Read the model definition and answer for the solid it produces. Units are mm, in the model's axes. Round coordinates to 2 decimals unless told otherwise and drop trailing zeros. Write each loop counter-clockwise with the first axis right and the second up, starting at its lowest first coordinate (ties: lowest second). Pieces come first, ordered by that corner, then holes. Notation, with made-up numbers: (62, 31.25) - (80, 31.25) arc R18 ccw to (80, 61.25) - close; hole circle Ø7 at (21, -8). An arc over 180 degrees is marked (long way). Use one line per item in the form item = value. Start each with the question number.
1) Consider line 1 along X through (y, z) = (65, 1); line 2 along X through (y, z) = (47, 3); line 3 along Z through (x, y) = (0, 52). Determine where each line is inside the solid, lowest interval first. Write a range as from..to.
2) The part is cut by section A-A, the plane z = 0. Give the vertices of the cut face in (x, y) (1 decimal), plus the area to 3 significant figures.
3) The part is cut by section C-C, the plane y = 31.5. Give the vertices of the cut face in (x, z), plus the area to 3 significant figures.
4) Each of these flat-tipped pins is pushed along its axis until it touches: pin 1 (1 mm diameter, centred on x = 0.5, y = 19.5, fed in from +Z); pin 2 (10 mm diameter, centred on y = 67, z = 0, fed in from +X); pin 3 (12 mm diameter, centred on x = -5, z = -5.5, fed in from +Y). Where does it stop, or does it pass through?
5) The part is cut by section B-B, the plane x = 0. Give the vertices of the cut face in (y, z) (1 decimal).
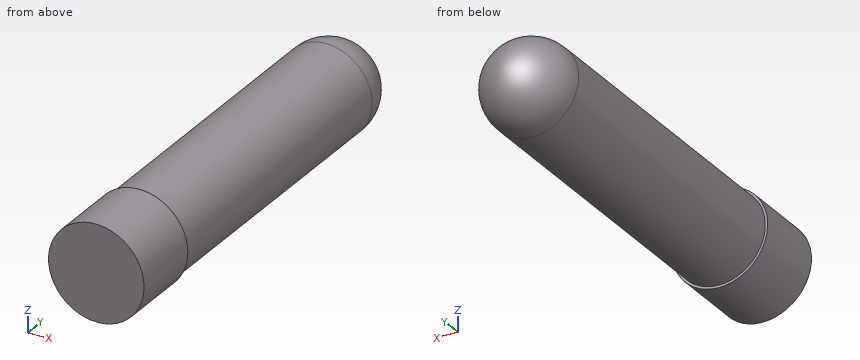
from build123d import *

# Parameters (mm, degrees)
SKETCH1_R           = 10
BOSS_EXTRUDE1_DEPTH = 15
BOSS_EXTRUDE3_START = -15
SKETCH3_R           = 9.5
BOSS_EXTRUDE3_DEPTH = 64
DOME1_FACE_RADIUS   = 9.5
DOME1_HEIGHT        = 10


with BuildPart() as part:
    # Sketch1 → Boss-Extrude1 (new body)
    with BuildSketch(Plane(origin=(0, 0, 0), x_dir=(1, 0, 0), z_dir=(0, 1, 0))):
        Circle(SKETCH1_R)
    extrude(amount=BOSS_EXTRUDE1_DEPTH)

    # Sketch3 → Boss-Extrude3 (add)
    with BuildSketch(Plane.XZ.offset(BOSS_EXTRUDE3_START)):
        Circle(SKETCH3_R)
    extrude(amount=-BOSS_EXTRUDE3_DEPTH)

    # Dome1: a dome of height H over a round flat face of radius A is a cap of a sphere of radius (A * A + H * H) / (2 * H)
    dome1_r = (DOME1_FACE_RADIUS * DOME1_FACE_RADIUS + DOME1_HEIGHT * DOME1_HEIGHT) / (2 * DOME1_HEIGHT)
    dome1_base = Plane((0, 79, 0), z_dir=(0, 1, 0))
    with Locations(dome1_base.offset(DOME1_HEIGHT - dome1_r)):
        dome1_ball = Sphere(dome1_r, mode=Mode.PRIVATE)
    add(split(dome1_ball, bisect_by=dome1_base, keep=Keep.TOP, mode=Mode.PRIVATE))


solid = part.part
Geometry results:
q1.line_1 = -9.45..9.45
q1.line_2 = -9.01..9.01
q1.line_3 = -9.5..9.5
q2.outline = (-10, 0) - (10, 0) - (10, 15) - (9.5, 15) - (9.5, 79) arc R9.5 ccw (long way) to (-9.5, 79) - (-9.5, 15) - (-10, 15) - close
q2.area = 1,670 mm2
q3.outline = circle Ø19 at (0, 0)
q3.area = 284 mm2
q4.pin_1 = 9.5
q4.pin_2 = 9.5
q4.pin_3 = 88.89
q5.outline = (0, -10) - (15, -10) - (15, -9.5) - (79, -9.5) arc R9.5 ccw (long way) to (79, 9.5) - (15, 9.5) - (15, 10) - (0, 10) - close
